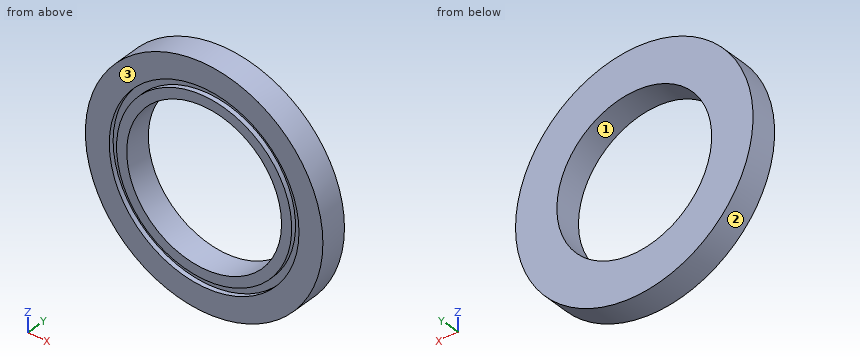
from build123d import *

# Parameters (mm, degrees)
F0_R     = 40
F0_R_2   = 26.075
F1_DEPTH = 9
F2_W     = 1.6
F2_H     = 2.45


with BuildPart() as f1:
    # F0 (on Front) → F1 (new body)
    with BuildSketch(Plane.XZ):
        Circle(F0_R)
        Circle(F0_R_2, mode=Mode.SUBTRACT)
    extrude(amount=F1_DEPTH)

    # F2 (on Right) → F3 (revolve, cut)
    with BuildSketch(Plane.YZ):
        with Locations((-8.2, -30.725)):
            Rectangle(F2_W, F2_H)
    revolve(axis=Axis((0, 0, 0), (0, 1, 0)), mode=Mode.SUBTRACT)


solid = f1.part
Geometry check sheet. Reference: the model listing, model coordinates, mm. Face numbers are marked on the shaded views. Give positions to 0.01 mm unless a question says otherwise; leave off trailing zeros. Write each loop counter-clockwise with the first axis right and the second up, starting at its lowest first coordinate (ties: lowest second). Pieces come first, ordered by that corner, then holes.
1) Go/stop test with flat-tipped pins: pin 1 Ø4 at (x, y) = (-13.5, -7) entering from +Z; pin 2 Ø3 at (y, z) = (-7.5, 21.5) entering from +X; pin 3 Ø12 at (x, z) = (12, 19) entering from -Y; pin 4 Ø3 at (x, y) = (28.5, -2) entering from -Z. Record where each tip stops, or that it passes through.
Values follow:
pin 1: stops at z = 38.31
pin 2: stops at x = 34.64
pin 3: stops at y = -9
pin 4: stops at z = -29.51
2) Cross-section at D-D (z = -33). Record the boundary of the cut face in (x, y), plus the area to 3 significant figures.
Values follow:
outline: (-22.61, -9) - (22.61, -9) - (22.61, 0) - (-22.61, 0) - close
area: 407 mm2
3) Cross-section at A-A (z = 0). Record the boundary of the cut face in (x, y) (3 decimals).
Values follow:
outline: (-40, -9) - (-31.95, -9) - (-31.95, -7.4) - (-29.5, -7.4) - (-29.5, -9) - (-26.075, -9) - (-26.075, 0) - (-40, 0) - close; (26.075, -9) - (29.5, -9) - (29.5, -7.4) - (31.95, -7.4) - (31.95, -9) - (40, -9) - (40, 0) - (26.075, 0) - close
4) Release check for a two-part mould opening along Z. For the marked faces 1, 2 and 3 record: released by +Z, released by -Z, zero draft, split by the parting line, or undercut.
Values follow:
face 1: undercut
face 2: split by the parting line
face 3: zero draft
5) Thickness scan on line 1 (Z direction, x = 0, y = -8.4) (3 decimals); line 2 (Z direction, x = 12.5, y = -8); line 3 (Z direction, x = 0, y = -2.75) (3 decimals). Record the ranges inside material, lowest first.
Values follow:
line 1: z = -40 to -31.95, -29.5 to -26.075, 26.075 to 29.5, 31.95 to 40
line 2: z = -38 to -29.4, -26.72 to -22.88, 22.88 to 26.72, 29.4 to 38
line 3: z = -40 to -26.075, 26.075 to 40
6) Cross-section at B-B (x = 0). Record the boundary of the cut face in (y, z) (3 decimals).
Values follow:
outline: (-9, -40) - (0, -40) - (0, -26.075) - (-9, -26.075) - (-9, -29.5) - (-7.4, -29.5) - (-7.4, -31.95) - (-9, -31.95) - close; (-9, 26.075) - (0, 26.075) - (0, 40) - (-9, 40) - (-9, 31.95) - (-7.4, 31.95) - (-7.4, 29.5) - (-9, 29.5) - close
7) Cross-section at C-C (y = -5). Record the boundary of the cut face in (x, z) (3 decimals), plus the area to 3 significant figures.
Values follow:
outline: circle Ø80 at (0, 0); hole circle Ø52.15 at (0, 0)
area: 2,890 mm2
